from build123d import *

# Parameters (mm, degrees)
F0_W      = 300
F0_H      = 210
F0_R      = 22.5
F1_DEPTH  = 40
F2_R      = 31
F2_R_2    = 22.5
F3_DEPTH  = 15
F4_R      = 36
F4_R_2    = 22.5
F5_DEPTH  = 21
F7_R      = 33
F8_DEPTH  = 2.5
F9_R      = 5
F10_DEPTH = 40
F11_SIZE  = 25
F12_R     = 5
F13_DEPTH = 12


with BuildPart() as f1:
    # F0 (on Top) → F1 (new body)
    with BuildSketch(Plane.XY):
        Rectangle(F0_W, F0_H)
        with Locations((-50, 0)):
            Circle(F0_R, mode=Mode.SUBTRACT)
        with Locations((50, 0)):
            Circle(F0_R, mode=Mode.SUBTRACT)
    extrude(amount=F1_DEPTH)

    # F2 (on face) → F3 (cut)
    with BuildSketch(Plane.XY.offset(40)):
        with Locations((-50, 0)):
            Circle(F2_R)
        with Locations((-50, 0)):
            Circle(F2_R_2, mode=Mode.SUBTRACT)
        with Locations((50, 0)):
            Circle(F2_R)
        with Locations((50, 0)):
            Circle(F2_R_2, mode=Mode.SUBTRACT)
    extrude(amount=-F3_DEPTH, mode=Mode.SUBTRACT)

    # F4 (on face) → F5 (cut)
    with BuildSketch(Plane(origin=(0, 0, 0), x_dir=(1, 0, 0), z_dir=(0, 0, -1))):
        with Locations((-50, 0)):
            Circle(F4_R)
        with Locations((-50, 0)):
            Circle(F4_R_2, mode=Mode.SUBTRACT)
        with Locations((50, 0)):
            Circle(F4_R)
        with Locations((50, 0)):
            Circle(F4_R_2, mode=Mode.SUBTRACT)
    extrude(amount=-F5_DEPTH, mode=Mode.SUBTRACT)

    # F7 (on offset) → F8 (cut)
    with BuildSketch(Plane.XY.offset(38.5)):
        with Locations((-50, 0)):
            Circle(F7_R)
        with Locations((50, 0)):
            Circle(F7_R)
    extrude(amount=-F8_DEPTH, mode=Mode.SUBTRACT)

    # F9 (on face) → F10 (cut)
    with BuildSketch(Plane.XY.offset(40)):
        with Locations((-140, 70)):
            Circle(F9_R)
        with Locations((140, -70)):
            Circle(F9_R)
    extrude(amount=-F10_DEPTH, mode=Mode.SUBTRACT)

    # F11
    f11_edges = [f1.edges().sort_by_distance(p)[0] for p in [
        (150, -105, 20),
        (-150, -105, 20),
        (150, 105, 20),
        (-150, 105, 20),
    ]]
    chamfer(f11_edges, length=F11_SIZE)

    # F12 (on face) → F13 (cut)
    with BuildSketch(Plane(origin=(0, 0, 0), x_dir=(1, 0, 0), z_dir=(0, 0, -1))):
        with Locations((120, 65)):
            Circle(F12_R)
        with Locations((-120, -65)):
            Circle(F12_R)
    extrude(amount=-F13_DEPTH, mode=Mode.SUBTRACT)


solid = f1.part
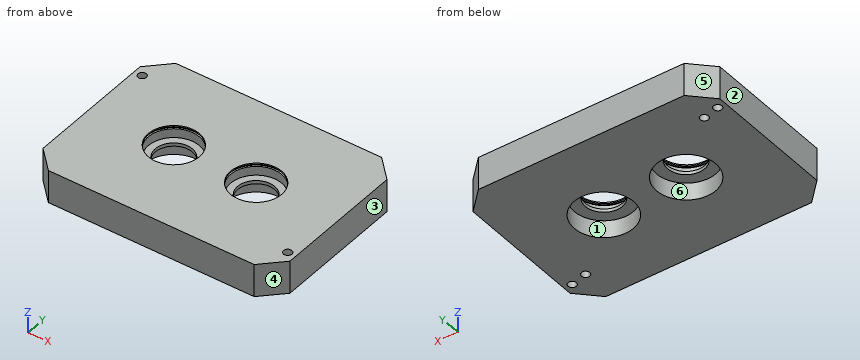
Verification items for the finished model (mm, model axes). Face numbers are marked on the shaded views. A direction names the side the tool comes from. Round coordinates to 2 decimals unless told otherwise and drop trailing zeros. Loops run counter-clockwise (first coordinate to the right, second up) from the corner with the lowest first, then second, coordinate; pieces in that order, holes last. Notation, with made-up numbers: (43, -27) - (100, -27) arc R30 ccw to (100, 12) - close; hole circle Ø8 at (11, -9). An arc over 180 degrees is marked (long way). Use a Markdown table: item, result. Add a question column.
1. Release check for a two-part mould opening along Y. For the marked faces 3, 4, 5 and 6 record: released by +Y, released by -Y, zero draft, split by the parting line, or undercut.
2. Access from +Z, -Z, +X, -X, +Y, -Y to the whole of each face (thin tool, end or side, straight path). Record for the marked faces 1 and 2.
3. Gauge pin test, flat ends, axial feed: pin 1 (18.5 mm diameter, centred on x = -38, y = 9, fed in from +Z); pin 2 (3 mm diameter, centred on x = -120.5, y = 64, fed in from -Z); pin 3 (20 mm diameter, centred on x = 50, y = 4.5, fed in from -Z). Record the tip position at first contact, or that the pin passes through.
4. Thickness scan on probe 1 along Y at (x, z) = (-50, 6); probe 2 along Y at (x, z) = (-50, 38.05); probe 3 along X at (y, z) = (0, 23). Record the ranges inside material, lowest first. Write a range as [from, to].
5. Section check B-B, the plane x = 64. Record the boundary of the cut face in (y, z).
6. Section check D-D, the plane y = 0. Give the number of separate pieces and of enclosed holes in the cut face, plus the area to 3 significant figures.
7. Section check C-C, the plane y = 85.5. Record the boundary of the cut face in (x, z), plus the area to 3 significant figures.
8. Section check A-A, the plane z = 16.5. Record the boundary of the cut face in (x, y), plus the area to 4 significant figures.
Checks:
| question | item | result |
|---|---|---|
| 1 | face 3 | zero draft |
| 1 | face 4 | released by -Y |
| 1 | face 5 | released by +Y |
| 1 | face 6 | undercut |
| 2 | face 1 | -Z |
| 2 | face 2 | +Z, -Z, -X, +Y, -Y |
| 3 | pin 1 | stops at z = 25 |
| 3 | pin 2 | stops at z = 12 |
| 3 | pin 3 | passes through |
| 4 | probe 1 | y = [-105, -36], [36, 105] |
| 4 | probe 2 | y = [-105, -33], [33, 105] |
| 4 | probe 3 | x = [-150, -72.5], [-27.5, 27.5], [72.5, 150] |
| 5 | outline | (-105, 0) - (-33.17, 0) - (-33.17, 21) - (-17.61, 21) - (-17.61, 25) - (-27.66, 25) - (-27.66, 36) - (-29.88, 36) - (-29.88, 38.5) - (-27.66, 38.5) - (-27.66, 40) - (-105, 40) - close; (17.61, 21) - (33.17, 21) - (33.17, 0) - (105, 0) - (105, 40) - (27.66, 40) - (27.66, 38.5) - (29.88, 38.5) - (29.88, 36) - (27.66, 36) - (27.66, 25) - (17.61, 25) - close |
| 6 | separate pieces | 3 |
| 6 | enclosed holes | 0 |
| 6 | area | 6,740 mm^2 |
| 7 | outline | (-144.5, 0) - (144.5, 0) - (144.5, 40) - (-144.5, 40) - close |
| 7 | area | 11,600 mm^2 |
| 8 | outline | (-150, -80) - (-125, -105) - (125, -105) - (150, -80) - (150, 80) - (125, 105) - (-125, 105) - (-150, 80) - close; hole circle Ø10 at (-140, 70); hole circle Ø72 at (-50, 0); hole circle Ø72 at (50, 0); hole circle Ø10 at (140, -70) |
| 8 | area | 53,450 mm^2 |
